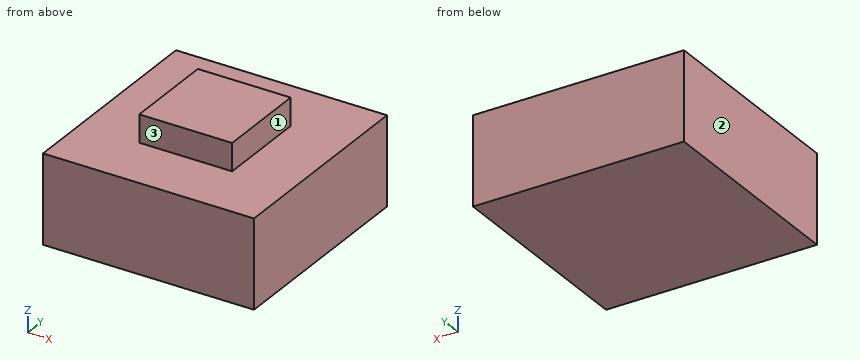
from build123d import *

# Parameters (mm, degrees)
F1_DEPTH = 44
F2_DEPTH = 72
F3_DEPTH = 28


with BuildPart() as f1:
    # F0 (on Front) → F1 (new body)
    with BuildSketch(Plane.XZ):
        Polygon((22, 13.045934), (0, 13.045934), (-22, 13.045934), (-22, 0), (22, 0), align=None)
    extrude(amount=F1_DEPTH)

    # F0 (on Front) → F2 (join)
    with BuildSketch(Plane.XZ):
        Polygon((50, 0), (22, 0), (-22, 0), (-50, 0), (-50, -41.984189), (0, -41.984189), (50, -41.984189), align=None)
    extrude(amount=F2_DEPTH)

    # F0 (on Front) → F3 (join)
    with BuildSketch(Plane.XZ):
        Polygon((50, 0), (22, 0), (-22, 0), (-50, 0), (-50, -41.984189), (0, -41.984189), (50, -41.984189), align=None)
    extrude(amount=-F3_DEPTH)


solid = f1.part
Geometry check sheet. Reference: the model listing, model coordinates, mm. Face numbers are marked on the shaded views. A direction names the side the tool comes from. Give positions to 0.01 mm unless a question says otherwise; leave off trailing zeros. Order: outer loops, then holes, each group sorted by start corner. A loop starts at its lowest first (then second) coordinate and runs counter-clockwise, first axis right, second up.
1. Sectioned sample at D-D (x = 35). Record the boundary of the cut face in (y, z).
Completed:
outline: (-72, -41.98) - (28, -41.98) - (28, 0) - (-72, 0) - close
2. Scan lines: line 1 (Z direction, x = 39, y = -56.5); line 2 (Y direction, x = -16.5, z = 4); line 3 (X direction, y = -18, z = 10.5). Record each from-to range of solid material in increasing order.
Completed:
line 1: z = -41.98 to 0
line 2: y = -44 to 0
line 3: x = -22 to 22
3. Sectioned sample at C-C (z = 3.5). Record the boundary of the cut face in (x, y), then the cut area to 3 significant figures.
Completed:
outline: (-22, -44) - (22, -44) - (22, 0) - (-22, 0) - close
area: 1,940 mm2
4. Sectioned sample at B-B (x = -17). Record the boundary of the cut face in (y, z), then the cut area to 3 significant figures.
Completed:
outline: (-72, -41.98) - (28, -41.98) - (28, 0) - (0, 0) - (0, 13.05) - (-44, 13.05) - (-44, 0) - (-72, 0) - close
area: 4,770 mm2
5. Depth check by flat-ended pin: pin 1 (4 mm diameter, centred on x = 6.5, z = 7.5, fed in from -Y); pin 2 (10.5 mm diameter, centred on y = -31.5, z = 5.5, fed in from -X); pin 3 (12 mm diameter, centred on x = 5.5, z = 1.5, fed in from -Y); pin 4 (10.5 mm diameter, centred on y = -12.5, z = 5.5, fed in from +X). Enter the tip coordinate at first touch or a pass-through.
Completed:
pin 1: stops at y = -44
pin 2: stops at x = -22
pin 3: stops at y = -72
pin 4: stops at x = 22
6. Access from +Z, -Z, +X, -X, +Y, -Y to the whole of each face (thin tool, end or side, straight path). Record for the marked faces 1, 2 and 3.
Completed:
face 1: +Z, +X, +Y, -Y
face 2: +Z, -Z, -X, +Y, -Y
face 3: +Z, +X, -X, -Y
7. Sectioned sample at A-A (y = -9.5). Record the boundary of the cut face in (x, z), then the cut area to 3 significant figures.
Completed:
outline: (-50, -41.98) - (50, -41.98) - (50, 0) - (22, 0) - (22, 13.05) - (-22, 13.05) - (-22, 0) - (-50, 0) - close
area: 4,770 mm2
